```python
from build123d import *

# Parameters (mm, degrees)
SKETCH2_W           = 103
SKETCH2_H           = 60
BOSS_EXTRUDE1_DEPTH = 6
SKETCH3_R           = 9.65
SKETCH3_R_2         = 2
BOSS_EXTRUDE2_DEPTH = 10
CUT_EXTRUDE1_DEPTH  = 2
SKETCH6_R           = 1
CUT_EXTRUDE2_DEPTH  = 120.804006757
SKETCH7_R           = 5.8
CUT_EXTRUDE3_DEPTH  = 0.2


with BuildPart() as part:
    # Sketch2 → Boss-Extrude1 (new body)
    with BuildSketch(Plane(origin=(0, 0, 0), x_dir=(1, 0, 0), z_dir=(0, 1, 0))):
        with Locations((51.5, 30)):
            Rectangle(SKETCH2_W, SKETCH2_H)
    extrude(amount=BOSS_EXTRUDE1_DEPTH)

    # Sketch3 → Boss-Extrude2 (add)
    # profile 1 of 5: a face of its own
    with BuildSketch(Plane(origin=(0, 6, 0), x_dir=(1, 0, 0), z_dir=(0, 1, 0))):
        with Locations(Location((78, 30, 0), (0, 0, 90))):
            Circle(SKETCH3_R)
    # profile 2 of 5: a face of its own
    with BuildSketch(Plane(origin=(0, 6, 0), x_dir=(1, 0, 0), z_dir=(0, 1, 0))):
        with BuildLine():
            Line((74, 55), (74, 50))
            ThreePointArc((74, 50), (78, 46), (82, 50))
            Line((82, 50), (82, 55))
            ThreePointArc((82, 55), (78, 59), (74, 55))
        make_face()
        with Locations(Location((78, 55, 0), (0, 0, 270))):
            Circle(SKETCH3_R_2, mode=Mode.SUBTRACT)
        with Locations(Location((78, 50, 0), (0, 0, 270))):
            Circle(SKETCH3_R_2, mode=Mode.SUBTRACT)
    # profile 3 of 5: a face of its own
    with BuildSketch(Plane(origin=(0, 6, 0), x_dir=(1, 0, 0), z_dir=(0, 1, 0))):
        with BuildLine():
            Line((74, 10), (74, 5))
            ThreePointArc((74, 5), (78, 1), (82, 5))
            Line((82, 5), (82, 10))
            ThreePointArc((82, 10), (78, 14), (74, 10))
        make_face()
        with Locations(Location((78, 10, 0), (0, 0, 270))):
            Circle(SKETCH3_R_2, mode=Mode.SUBTRACT)
        with Locations(Location((78, 5, 0), (0, 0, 270))):
            Circle(SKETCH3_R_2, mode=Mode.SUBTRACT)
    # profile 4 of 5: a face of its own
    with BuildSketch(Plane(origin=(0, 6, 0), x_dir=(1, 0, 0), z_dir=(0, 1, 0))):
        with BuildLine():
            ThreePointArc((28.84758707, 8.766166365), (23.953123955, 3.150764937), (31.359338334, 3.948568773))
            add(Edge.make_bspline(
                [(31.359338334, 3.948568773), (32.83524335, 6.912030452), (36.017562261, 6.146478651)],
                knots=[0, 0, 0, 1, 1, 1], degree=2))
            ThreePointArc((36.017562261, 6.146478651), (40.636992833, 11.849235063), (33.316625669, 11.326938122))
            add(Edge.make_bspline(
                [(28.84758707, 8.766166365), (32.122274454, 8.279521447), (33.316625669, 11.326938122)],
                knots=[0, 0, 0, 1, 1, 1], degree=2))
        make_face()
        with Locations(Location((37.090116788, 10, 0), (0, 0, 270))):
            Circle(SKETCH3_R_2, mode=Mode.SUBTRACT)
        with Locations(Location((27.5, 5, 0), (0, 0, 270))):
            Circle(SKETCH3_R_2, mode=Mode.SUBTRACT)
    # profile 5 of 5: a face of its own
    with BuildSketch(Plane(origin=(0, 6, 0), x_dir=(1, 0, 0), z_dir=(0, 1, 0))):
        with BuildLine():
            add(Edge.make_bspline(
                [(31.355779837, 56.064406805), (32.362019475, 52.752034899), (35.895571064, 53.817467814)],
                knots=[0.017920477, 0.017920477, 0.017920477, 1, 1, 1], degree=2))
            add(Edge.make_bspline(
                [(31.319898681, 56.18674937), (31.337418499, 56.124849248), (31.355779837, 56.064406805)],
                knots=[0, 0, 0, 0.017920477, 0.017920477, 0.017920477], degree=2))
            ThreePointArc((31.319898681, 56.18674937), (23.953123955, 56.849235063), (28.714062153, 51.188694044))
            add(Edge.make_bspline(
                [(28.714062153, 51.188694044), (28.774843392, 51.209770338), (28.83491132, 51.229322108)],
                knots=[0, 0, 0, 0.017920477, 0.017920477, 0.017920477], degree=2))
            add(Edge.make_bspline(
                [(28.83491132, 51.229322108), (32.126759022, 52.300799854), (33.276340108, 48.793721661)],
                knots=[0.017920477, 0.017920477, 0.017920477, 1, 1, 1], degree=2))
            ThreePointArc((33.276340108, 48.793721661), (40.636992833, 48.150764937), (35.895571064, 53.817467814))
        make_face()
        with Locations(Location((37.090116788, 50, 0), (0, 0, 270))):
            Circle(SKETCH3_R_2, mode=Mode.SUBTRACT)
        with Locations(Location((27.5, 55, 0), (0, 0, 270))):
            Circle(SKETCH3_R_2, mode=Mode.SUBTRACT)
    extrude(amount=BOSS_EXTRUDE2_DEPTH)

    # Sketch5 → Cut-Extrude1 (cut)
    with BuildSketch(Plane(origin=(0, 6, 0), x_dir=(1, 0, 0), z_dir=(0, 1, 0))):
        with BuildLine():
            Line((9, 0), (0, 0))
            Line((0, 0), (0, 9))
            Line((0, 9), (4, 9))
            ThreePointArc((4, 9), (7.535533906, 7.535533906), (9, 4))
            Line((9, 4), (9, 0))
        make_face()
        with BuildLine():
            Line((0, 60), (0, 51))
            Line((0, 51), (4, 51))
            ThreePointArc((4, 51), (7.535533906, 52.464466094), (9, 56))
            Line((9, 56), (9, 60))
            Line((9, 60), (0, 60))
        make_face()
        with BuildLine():
            Line((94, 60), (103, 60))
            Line((103, 60), (103, 51))
            Line((103, 51), (99, 51))
            ThreePointArc((99, 51), (95.464466094, 52.464466094), (94, 56))
            Line((94, 56), (94, 60))
        make_face()
        with BuildLine():
            Line((103, 0), (103, 9))
            Line((103, 9), (99, 9))
            ThreePointArc((99, 9), (95.464466094, 7.535533906), (94, 4))
            Line((94, 4), (94, 0))
            Line((94, 0), (103, 0))
        make_face()
    extrude(amount=-CUT_EXTRUDE1_DEPTH, mode=Mode.SUBTRACT)

    # Sketch6 → Cut-Extrude2 (cut, through all)
    with BuildSketch(Plane(origin=(0, 4, 0), x_dir=(1, 0, 0), z_dir=(0, 1, 0))):
        with Locations(Location((4, 4, 0), (0, 0, 270))):
            Circle(SKETCH6_R)
        with Locations(Location((4, 56, 0), (0, 0, 270))):
            Circle(SKETCH6_R)
        with Locations(Location((99, 56, 0), (0, 0, 270))):
            Circle(SKETCH6_R)
        with Locations(Location((99, 4, 0), (0, 0, 270))):
            Circle(SKETCH6_R)
    extrude(amount=-CUT_EXTRUDE2_DEPTH, mode=Mode.SUBTRACT)

    # Sketch7 → Cut-Extrude3 (cut)
    with BuildSketch(Plane(origin=(0, 16, 0), x_dir=(1, 0, 0), z_dir=(0, 1, 0))):
        with Locations(Location((78, 30, 0), (0, 0, 270))):
            Circle(SKETCH7_R)
    extrude(amount=-CUT_EXTRUDE3_DEPTH, mode=Mode.SUBTRACT)


solid = part.part
```
Geometry check sheet. Reference: the model listing, model coordinates, mm. A direction names the side the tool comes from. Give positions to 0.01 mm unless a question says otherwise; leave off trailing zeros. Write each loop counter-clockwise with the first axis right and the second up, starting at its lowest first coordinate (ties: lowest second). Pieces come first, ordered by that corner, then holes. Notation, with made-up numbers: (43, 28.5) - (53, 28.5) arc R13 cw to (53, 32.5) - close; hole circle Ø11 at (32.25, -30). An arc over 180 degrees is marked (long way). Use a Markdown table: item, result.
Q1. Section check C-C, the plane z = -27. Enter the section's corners in (x, y).
Computed:
| item | result |
|---|---|
| outline | (0, 0) - (103, 0) - (103, 6) - (87.17, 6) - (87.17, 16) - (82.96, 16) - (82.96, 15.8) - (73.04, 15.8) - (73.04, 16) - (68.83, 16) - (68.83, 6) - (0, 6) - close |
Q2. Draft check along X on faces 1 (the face through (9, 5, -58)), 2 (the face through (84, 16, -30)), 3 (the face through (4.676, 2.028, -4.737)), 4 (the face through (75.101, 10.93, -39.204)). Enter one of: pulls with the +X half, pulls with the -X half, needs draft (parallel to the pull), parting line crosses it, or undercut.
Computed:
| item | result |
|---|---|
| face 1 | pulls with the -X half |
| face 2 | needs draft |
| face 3 | undercut |
| face 4 | parting line crosses it |
Q3. Set-up check for faces 5 (the face through (5.4, 4, -55.6)), 6 (the face through (24.02, 10.93, -56.97)), 7 (the face through (78, 11, -59)), 8 (the face through (96, 5, -52)), 9 (the face through (9, 5, -2)): record each of +Z, -Z, +X, -X, +Y, -Y from which the full face is reachable in a straight line by a thin tool's end or side.
Computed:
| item | result |
|---|---|
| face 5 | -Z, -X, +Y |
| face 6 | +Y |
| face 7 | -Z, +Y |
| face 8 | -Z, +X, +Y |
| face 9 | +Z, -X, +Y |
Q4. Go/stop test with flat-tipped pins: P1, Ø0.6, axis at x = 102, y = 5, coming from the +Z side; P2, Ø8, axis at x = 12.5, z = -44.5, coming from the +Y side; P3, Ø4, axis at x = 85.5, y = 10.5, coming from the -Z side; P4, Ø5, axis at y = 12, z = -42.5, coming from the +X side. Record where each tip stops, or that it passes through.
Computed:
| item | result |
|---|---|
| P1 | stops at z = -9 |
| P2 | stops at y = 6 |
| P3 | stops at z = -37.93 |
| P4 | passes through |
Q5. Section check A-A, the plane x = 95. Enter the section's corners in (y, z), then the cut area to 3 significant figures.
Computed:
| item | result |
|---|---|
| outline | (0, -60) - (4, -60) - (4, -53) - (6, -53) - (6, -7) - (4, -7) - (4, 0) - (0, 0) - close |
| area | 332 mm² |
Q6. Section check D-D, the plane x = 70. Enter the section's corners in (y, z), then the cut area to 3 significant figures.
Computed:
| item | result |
|---|---|
| outline | (0, -60) - (6, -60) - (6, -35.4) - (16, -35.4) - (16, -24.6) - (6, -24.6) - (6, 0) - (0, 0) - close |
| area | 468 mm² |
Q7. Section check B-B, the plane y = 7.5. Give the number of separate pieces and of enclosed holes in the cut face, then the cut area to 3 significant figures.
Computed:
| item | result |
|---|---|
| separate pieces | 5 |
| enclosed holes | 8 |
| area | 598 mm² |
Q8. Thickness scan on L1, parallel to X at y = 1, z = -56; L2, parallel to X at y = 13, z = -55; L3, parallel to Z at x = 38, y = 14.5. Record the ranges inside material, lowest first. Write a range as [from, to].
Computed:
| item | result |
|---|---|
| L1 | x = [0, 3], [5, 98], [100, 103] |
| L2 | x = [23.5, 25.5], [29.5, 31.81], [74, 76], [80, 82] |
| L3 | z = [-53.9, -51.78], [-48.22, -46.1], [-13.9, -11.78], [-8.22, -6.1] |
